Check sheet for the modelled part. Datum: model origin and axes. Units: mm. A direction names the side the tool comes from. Give positions to 0.01 mm unless a question says otherwise; leave off trailing zeros. Order: outer loops, then holes, each group sorted by start corner. A loop starts at its lowest first (then second) coordinate and runs counter-clockwise, first axis right, second up.
Item 1: Sectioned sample at C-C on x = 34.5. Record the boundary of the cut face in (y, z), and give its area (3 significant figures).
Item 2: Gauge pin test, flat ends, axial feed: P1, Ø6, axis at x = 5, z = -39.5, coming from the -Y side; P2, Ø3, axis at x = -18, y = -90.5, coming from the -Z side; P3, Ø2, axis at x = 6, y = -61.5, coming from the -Z side. Record the tip position at first contact, or that the pin passes through.
Item 3: Sectioned sample at D-D on y = -120. Record the boundary of the cut face in (x, z).
Item 4: Material ranges on line 1 along Y through (x, z) = (-23, -27.5); line 2 along X through (y, z) = (-65.5, -1); line 3 along X through (y, z) = (-83, 5), recorded low to high.
Item 5: Sectioned sample at B-B on y = -37.5. Record the boundary of the cut face in (x, z), and give its area (3 significant figures).
Item 6: Sectioned sample at A-A on z = 0. Record the boundary of the cut face in (x, y), and give its area (3 significant figures).
Item 7: Access from +Z, -Z, +X, -X, +Y, -Y to the whole of each face (thin tool, end or side, straight path). Record for faces 1 (the flat face through (46.08, -10, 0)), 2 (the cylindrical face through (24.93, -34.21, 7.85)).
from build123d import *

# Parameters (mm, degrees)
F1_DEPTH = 20.5
F2_R     = 26.136981888
F3_DEPTH = 32.8
F4_SIZE  = 5
F5_DEPTH = 102.9
F6_SIZE  = 5


with BuildPart() as f1:
    # F0 (on Front) → F1 (new body)
    with BuildSketch(Plane.XZ):
        Polygon((46.0798591375, -26.6042190773), (46.0798591375, 26.6042190773), (0, 53.2084381546), (-46.0798591375, 26.6042190773), (-46.0798591375, -26.6042190773), (0, -53.2084381546), align=None)
    extrude(amount=F1_DEPTH)

    # F2 (on face) → F3 (join)
    with BuildSketch(Plane.XZ.offset(20.5)):
        Circle(F2_R)
    extrude(amount=F3_DEPTH)

    # F4
    f4_edges = [f1.edges().sort_by_distance(p)[0] for p in [
        (-26.136982, -53.3, 0),
    ]]
    chamfer(f4_edges, length=F4_SIZE)

    # F5 (add): a face of the model
    f5_faces = [f1.faces().sort_by_distance(p)[0] for p in [
        (0, -53.3, 0),
    ]]
    extrude(f5_faces, amount=F5_DEPTH)

    # F6
    f6_edges = [f1.edges().sort_by_distance(p)[0] for p in [
        (-21.136982, -156.2, 0),
    ]]
    chamfer(f6_edges, length=F6_SIZE)


solid = f1.part
Report:
1. outline: (-20.5, -33.29) - (0, -33.29) - (0, 33.29) - (-20.5, 33.29) - close
1. area: 1,360 mm2
2. P1: stops at y = -20.5
2. P2: stops at z = -13.21
2. P3: stops at z = -20.54
3. outline: circle Ø42.27 at (0, 0)
4. line 1: y = -20.5 to 0
4. line 2: x = -21.11 to 21.11
4. line 3: x = -20.54 to 20.54
5. outline: circle Ø52.27 at (0, 0)
5. area: 2,150 mm2
6. outline: (-46.08, -20.5) - (-26.14, -20.5) - (-26.14, -48.3) - (-21.14, -53.3) - (-21.14, -151.2) - (-16.14, -156.2) - (16.14, -156.2) - (21.14, -151.2) - (21.14, -53.3) - (26.14, -48.3) - (26.14, -20.5) - (46.08, -20.5) - (46.08, 0) - (-46.08, 0) - close
6. area: 7,900 mm2
7. face 1: +Z, -Z, +X, +Y, -Y
7. face 2: -Y
